Part model, mm, in its own coordinate system. Face numbers are marked on the shaded views. A direction names the side the tool comes from. Round coordinates to 2 decimals unless told otherwise and drop trailing zeros. Loops run counter-clockwise (first coordinate to the right, second up) from the corner with the lowest first, then second, coordinate; pieces in that order, holes last.
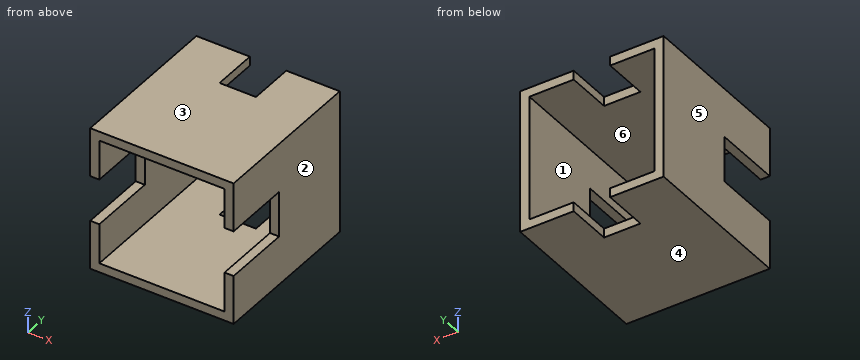
from build123d import *

# Parameters (mm, degrees)
SKETCH1_W           = 31.5
SKETCH1_H           = 31.5
SKETCH1_W_2         = 27.5
SKETCH1_H_2         = 27.5
BOSS_EXTRUDE1_DEPTH = 35
SKETCH2_W           = 10
SKETCH2_H           = 15
CUT_EXTRUDE1_DEPTH  = 32.5
SKETCH3_W           = 8
SKETCH3_H           = 10
CUT_EXTRUDE2_DEPTH  = 32.5


with BuildPart() as part:
    # Sketch1 → Boss-Extrude1 (new body)
    with BuildSketch(Plane(origin=(0, 0, 0), x_dir=(1, 0, 0), z_dir=(0, 1, 0))):
        Rectangle(SKETCH1_W, SKETCH1_H)
        Rectangle(SKETCH1_W_2, SKETCH1_H_2, mode=Mode.SUBTRACT)
    extrude(amount=BOSS_EXTRUDE1_DEPTH)

    # Sketch2 → Cut-Extrude1 (cut, through all)
    with BuildSketch(Plane(origin=(15.75, 0, 0), x_dir=(0, 0, -1), z_dir=(1, 0, 0))):
        with Locations((0, 7.5)):
            Rectangle(SKETCH2_W, SKETCH2_H)
    extrude(amount=-CUT_EXTRUDE1_DEPTH, mode=Mode.SUBTRACT)

    # Sketch3 → Cut-Extrude2 (cut, through all)
    with BuildSketch(Plane(origin=(0, 0, -15.75), x_dir=(-1, 0, 0), z_dir=(0, 0, -1))):
        with Locations((0, 30)):
            Rectangle(SKETCH3_W, SKETCH3_H)
    extrude(amount=-CUT_EXTRUDE2_DEPTH, mode=Mode.SUBTRACT)


solid = part.part
1) Slice it at A-A, the plane z = 4.5. Give the cut face in (x, y).
Values:
outline: (-15.75, 15) - (-13.75, 15) - (-13.75, 35) - (-15.75, 35) - close; (13.75, 15) - (15.75, 15) - (15.75, 35) - (13.75, 35) - close
2) Tool access for the marked faces 5 and 6: list every direction of +Z, -Z, +X, -X, +Y, -Y with a clear straight run to the whole face (end or side of a thin tool).
Values:
face 5: +Z, -Z, -X, +Y, -Y
face 6: +Y, -Y
3) Drop flat-ended pins along their axis: pin 1 Ø3 at (x, z) = (12.5, -1.5) entering from -Y; pin 2 Ø0.6 at (x, z) = (-0.5, -14.5) entering from +Y. Give the stop position or say it passes through.
Values:
pin 1: stops at y = 15
pin 2: stops at y = 25
4) Wall check: line 1 along Z through (x, y) = (-12.5, 23). Give the ranges that are in metal, low to high.
Values:
line 1: z = -15.75 to -13.75, 13.75 to 15.75
5) Slice it at B-B, the plane x = 1.5. Give the cut face in (y, z).
Values:
outline: (0, -15.75) - (25, -15.75) - (25, -13.75) - (0, -13.75) - close; (0, 13.75) - (25, 13.75) - (25, 15.75) - (0, 15.75) - close
6) Slice it at D-D, the plane y = 32.5. Give the cut face in (x, z).
Values:
outline: (-15.75, -15.75) - (-4, -15.75) - (-4, -13.75) - (-13.75, -13.75) - (-13.75, 13.75) - (-4, 13.75) - (-4, 15.75) - (-15.75, 15.75) - close; (4, -15.75) - (15.75, -15.75) - (15.75, 15.75) - (4, 15.75) - (4, 13.75) - (13.75, 13.75) - (13.75, -13.75) - (4, -13.75) - close
7) Mould opens along Z. For the marked faces 1, 2, 3 and 4 say: released by +Z, released by -Z, zero draft, split by the parting line, or undercut.
Values:
face 1: undercut
face 2: zero draft
face 3: released by +Z
face 4: released by -Z
8) Slice it at C-C, the plane y = 14.5. Give the cut face in (x, z), then the cut area to 3 significant figures.
Values:
outline: (-15.75, -15.75) - (15.75, -15.75) - (15.75, -5) - (13.75, -5) - (13.75, -13.75) - (-13.75, -13.75) - (-13.75, -5) - (-15.75, -5) - close; (-15.75, 5) - (-13.75, 5) - (-13.75, 13.75) - (13.75, 13.75) - (13.75, 5) - (15.75, 5) - (15.75, 15.75) - (-15.75, 15.75) - close
area: 196 mm2
